The model under review builds one solid part; all positions refer to its coordinate system, in mm. Coordinates: 2 decimals unless noted, no trailing zeros. Write each loop counter-clockwise with the first axis right and the second up, starting at its lowest first coordinate (ties: lowest second). Pieces come first, ordered by that corner, then holes.
```python
from build123d import *

# Parameters (mm, degrees)
F0_W     = 260
F0_H     = 320
F1_DEPTH = 10
F2_R     = 20
F4_DEPTH = 14


with BuildPart() as f1:
    # F0 (on Front) → F1 (new body)
    with BuildSketch(Plane.XZ):
        Rectangle(F0_W, F0_H)
    extrude(amount=F1_DEPTH)

    # F2
    f2_edges = [f1.edges().sort_by_distance(p)[0] for p in [
        (-130, -5, 160),
        (130, -5, 160),
    ]]
    fillet(f2_edges, radius=F2_R)

    # F3 (on face) → F4 (join)
    with BuildSketch(Plane(origin=(0, 0, 0), x_dir=(-1, 0, 0), z_dir=(0, 1, 0))):
        with BuildLine():
            ThreePointArc((-97.5, -120), (-105, -112.5), (-112.5, -120))
            Line((-112.5, -120), (-105, -120))
            Line((-105, -120), (-105, -127.5))
            ThreePointArc((-105, -127.5), (-99.696699, -125.303301), (-97.5, -120))
        make_face()
        with BuildLine():
            Line((-105, -120), (-112.5, -120))
            ThreePointArc((-112.5, -120), (-110.303301, -125.303301), (-105, -127.5))
            Line((-105, -127.5), (-105, -120))
        make_face()
        with BuildLine():
            ThreePointArc((105, -127.5), (110.303301, -125.303301), (112.5, -120))
            Line((112.5, -120), (105, -120))
            Line((105, -120), (105, -127.5))
        make_face()
        with BuildLine():
            Line((105, -120), (112.5, -120))
            ThreePointArc((112.5, -120), (99.696699, -114.696699), (105, -127.5))
            Line((105, -127.5), (105, -120))
        make_face()
        with BuildLine():
            ThreePointArc((105, 127.5), (99.696699, 114.696699), (112.5, 120))
            Line((112.5, 120), (105, 120))
            Line((105, 120), (105, 127.5))
        make_face()
        with BuildLine():
            Line((105, 120), (112.5, 120))
            ThreePointArc((112.5, 120), (110.303301, 125.303301), (105, 127.5))
            Line((105, 127.5), (105, 120))
        make_face()
        with BuildLine():
            ThreePointArc((-105, 127.5), (-110.303301, 125.303301), (-112.5, 120))
            Line((-112.5, 120), (-105, 120))
            Line((-105, 120), (-105, 127.5))
        make_face()
        with BuildLine():
            Line((-105, 120), (-112.5, 120))
            ThreePointArc((-112.5, 120), (-105, 112.5), (-97.5, 120))
            ThreePointArc((-97.5, 120), (-99.696699, 125.303301), (-105, 127.5))
            Line((-105, 127.5), (-105, 120))
        make_face()
    extrude(amount=F4_DEPTH)


solid = f1.part
```
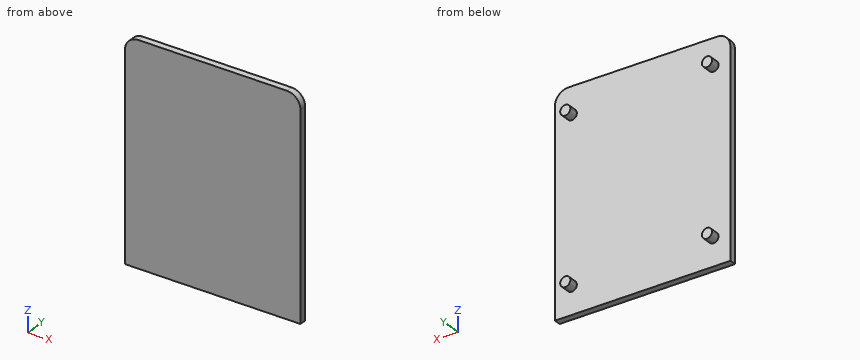
Item 1: Take a section at B-B, the plane x = -101. Write out the cut boundary in (y, z), plus the area to 3 significant figures.
Solved:
outline: (-10, -160) - (0, -160) - (0, -126.34) - (14, -126.34) - (14, -113.66) - (0, -113.66) - (0, 113.66) - (14, 113.66) - (14, 126.34) - (0, 126.34) - (0, 160) - (-10, 160) - close
area: 3,560 mm2
Item 2: Take a section at C-C, the plane x = 68.5. Write out the cut boundary in (y, z).
Solved:
outline: (-10, -160) - (0, -160) - (0, 160) - (-10, 160) - close
Item 3: Take a section at A-A, the plane z = -100. Write out the cut boundary in (x, y).
Solved:
outline: (-130, -10) - (130, -10) - (130, 0) - (-130, 0) - close
Item 4: For pin 1 (3 mm diameter, centred on x = 6, z = -86, fed in from +Y), flat-tipped, find the tip position at first contact; note if it passes through.
Solved:
pin 1: stops at y = 0
Item 5: To check wall thickness, follow line 1 along Y through (x, z) = (1, -60); line 2 along Z through (x, y) = (-105.5, 7.5); line 3 along Z through (x, y) = (-101, 3.5). State the ranges of each line that lie inside material, in increasing order.
Solved:
line 1: y = -10 to 0
line 2: z = -127.48 to -112.52, 112.52 to 127.48
line 3: z = -126.34 to -113.66, 113.66 to 126.34
